```python
from build123d import *

# Parameters (mm, degrees)
BOSS_EXTRUDE1_DEPTH   = 8
CIRPATTERN1_COUNT     = 2
SKETCH3_R             = 12
CUT_EXTRUDE1_DEPTH    = 95.051900566
CUT_EXTRUDE2_START    = -2.6
CUT_EXTRUDE2_DEPTH    = 97.651900566
M3_CLEARANCE_HOLE1_D  = 3.4
CIRPATTERN2_COUNT     = 6
CIRPATTERN3_START     = 22
CIRPATTERN3_OUTLINE_R = 12
CIRPATTERN3_DEPTH     = 8
CUT_EXTRUDE3_DEPTH    = 3.6
M3_CLEARANCE_HOLE2_D  = 3.4
CIRPATTERN4_COUNT     = 6
SKETCH15_W            = 0.975112204
SKETCH15_H            = 3.233161508
CUT_EXTRUDE4_DEPTH    = 2.6
CIRPATTERN5_COUNT     = 3
CIRPATTERN5_ANGLE     = 120


# Read off the part's stored shape, not the designer's step: CSK for M3 Hex Socket Countersunk Cap Screw1, CirPattern3
with BuildPart() as part:
    # Sketch1 → Boss-Extrude1 (new body)
    with BuildSketch(Plane(origin=(0, 0, 0), x_dir=(1, 0, 0), z_dir=(0, 1, 0))):
        with BuildLine():
            Line((21.213203436, -21.213203436), (12.426406871, -30))
            Line((12.426406871, -30), (-54.826406871, -30))
            Line((-54.826406871, -30), (-54.826406871, -22))
            Line((-54.826406871, -22), (-23.763220436, 18.311454189))
            ThreePointArc((-23.763220436, 18.311454189), (19.803416038, 22.534966457), (21.213203436, -21.213203436))
        make_face()
    boss_extrude1 = extrude(amount=BOSS_EXTRUDE1_DEPTH)

    # CirPattern1: Boss-Extrude1 ×2 about axis
    cirpattern1_axis = Axis((-21.2, 15, 15), (0, 0.7071067811865476, -0.7071067811865476))
    for i in range(1, CIRPATTERN1_COUNT):
        add(boss_extrude1.rotate(cirpattern1_axis, i * 360 / CIRPATTERN1_COUNT))

    # Sketch3 → Cut-Extrude1 (cut, through all)
    with BuildSketch(Plane(origin=(0, 8, 0), x_dir=(1, 0, 0), z_dir=(0, 1, 0))):
        with Locations(Location((0, 0, 0), (0, 0, 270))):
            Circle(SKETCH3_R)
    extrude(amount=-CUT_EXTRUDE1_DEPTH, mode=Mode.SUBTRACT)

    # Sketch4 → Cut-Extrude2 (cut)
    with BuildSketch(Plane(origin=(0, 8, 0), x_dir=(1, 0, 0), z_dir=(0, 1, 0)).offset(CUT_EXTRUDE2_START)):
        Polygon((27, 3.233161507), (24.2, 1.616580754), (24.2, -1.616580754), (27, -3.233161507), (29.8, -1.616580754), (29.8, 1.616580754), align=None)
    cut_extrude2 = extrude(amount=CUT_EXTRUDE2_DEPTH, mode=Mode.SUBTRACT)

    # M3 Clearance Hole1 (through all)
    with Locations(Plane(origin=(0, 5.4, 0), x_dir=(1, 0, 0), z_dir=(0, 1, 0))):
        with Locations((27, 0)):
            m3_clearance_hole1 = Hole(M3_CLEARANCE_HOLE1_D / 2)

    # CirPattern2: Cut-Extrude2, M3 Clearance Hole1 ×6 about axis
    cirpattern2_axis = Axis((0, 0, 0), (0, 1, 0))
    add([cut_extrude2.rotate(cirpattern2_axis, i * 360 / CIRPATTERN2_COUNT) for i in range(1, CIRPATTERN2_COUNT)], mode=Mode.SUBTRACT)
    add([m3_clearance_hole1.rotate(cirpattern2_axis, i * 360 / CIRPATTERN2_COUNT) for i in range(1, CIRPATTERN2_COUNT)], mode=Mode.SUBTRACT)

    # CSK for M3 Hex Socket Countersunk Ca 2 → CSK for M3 Hex Socket Countersunk Cap Screw1 (revolve, cut)
    with BuildSketch(Plane(origin=(-15.5, 0, -15.5), x_dir=(1, 0, 0), z_dir=(0, 0, 1))):
        Polygon((1.8, 1.56), (1.8, 8), (0, 8), (0, 0), (3.36, 0), align=None)
    revolve(axis=Axis((-15.5, 0, -15.5), (0, 1, 0)), mode=Mode.SUBTRACT)

    # CSK for M3 Hex Socket Countersunk Ca 3 o → CSK for M3 Hex Socket Countersunk Ca 3 (revolve, cut)
    with BuildSketch(Plane(origin=(15.5, 0, 15.5), x_dir=(1, 0, 0), z_dir=(0, 0, 1))):
        Polygon((1.8, 1.56), (1.8, 8), (0, 8), (0, 0), (3.36, 0), align=None)
    revolve(axis=Axis((15.5, 0, 15.5), (0, 1, 0)), mode=Mode.SUBTRACT)

    # CSK for M3 Hex Socket Countersunk Ca 4 o → CSK for M3 Hex Socket Countersunk Ca 4 (revolve, cut)
    with BuildSketch(Plane(origin=(-15.5, 0, 15.5), x_dir=(1, 0, 0), z_dir=(0, 0, 1))):
        Polygon((1.8, 1.56), (1.8, 8), (0, 8), (0, 0), (3.36, 0), align=None)
    revolve(axis=Axis((-15.5, 0, 15.5), (0, 1, 0)), mode=Mode.SUBTRACT)

    # CSK for M3 Hex Socket Countersunk Ca 5 o → CSK for M3 Hex Socket Countersunk Ca 5 (revolve, cut)
    with BuildSketch(Plane(origin=(15.5, 0, -15.5), x_dir=(1, 0, 0), z_dir=(0, 0, 1))):
        Polygon((1.8, 1.56), (1.8, 8), (0, 8), (0, 0), (3.36, 0), align=None)
    revolve(axis=Axis((15.5, 0, -15.5), (0, 1, 0)), mode=Mode.SUBTRACT)

    # CirPattern3 outline → CirPattern3 (cut)
    with BuildSketch(Plane.XY.offset(CIRPATTERN3_START)):
        with Locations((-42.4, 30)):
            Circle(CIRPATTERN3_OUTLINE_R)
    extrude(amount=CIRPATTERN3_DEPTH, mode=Mode.SUBTRACT)

    # CirPattern3 2 outline → CirPattern3 2 (revolve, cut)
    with BuildSketch(Plane(origin=(-26.9, 45.5, 0), x_dir=(1, 0, 0), z_dir=(0, -1, 0))):
        Polygon((0, 22), (1.8, 22), (1.8, 28.44), (3.36, 30), (0, 30), align=None)
    revolve(axis=Axis((-26.9, 45.5, 0), (0, 0, 1)), mode=Mode.SUBTRACT)

    # CirPattern3 3 outline → CirPattern3 3 (revolve, cut)
    with BuildSketch(Plane(origin=(-57.9, 14.5, 0), x_dir=(1, 0, 0), z_dir=(0, -1, 0))):
        Polygon((0, 22), (1.8, 22), (1.8, 28.44), (3.36, 30), (0, 30), align=None)
    revolve(axis=Axis((-57.9, 14.5, 0), (0, 0, 1)), mode=Mode.SUBTRACT)

    # CirPattern3 4 outline → CirPattern3 4 (revolve, cut)
    with BuildSketch(Plane(origin=(-26.9, 14.5, 0), x_dir=(1, 0, 0), z_dir=(0, -1, 0))):
        Polygon((0, 22), (1.8, 22), (1.8, 28.44), (3.36, 30), (0, 30), align=None)
    revolve(axis=Axis((-26.9, 14.5, 0), (0, 0, 1)), mode=Mode.SUBTRACT)

    # CirPattern3 5 outline → CirPattern3 5 (revolve, cut)
    with BuildSketch(Plane(origin=(-57.9, 45.5, 0), x_dir=(1, 0, 0), z_dir=(0, -1, 0))):
        Polygon((0, 22), (1.8, 22), (1.8, 28.44), (3.36, 30), (0, 30), align=None)
    revolve(axis=Axis((-57.9, 45.5, 0), (0, 0, 1)), mode=Mode.SUBTRACT)

    # Sketch11 → Cut-Extrude3 (cut)
    with BuildSketch(Plane(origin=(0, 0, 22), x_dir=(-1, 0, 0), z_dir=(0, 0, -1))):
        Polygon((45.633161507, 46), (44.016580754, 48.8), (40.783419246, 48.8), (39.166838493, 46), (40.783419246, 43.2), (44.016580754, 43.2), align=None)
    cut_extrude3 = extrude(amount=-CUT_EXTRUDE3_DEPTH, mode=Mode.SUBTRACT)

    # M3 Clearance Hole2 (through all)
    with Locations(Plane(origin=(0, 0, 25.6), x_dir=(-1, 0, 0), z_dir=(0, 0, -1))):
        with Locations((42.4, 46)):
            m3_clearance_hole2 = Hole(M3_CLEARANCE_HOLE2_D / 2)

    # CirPattern4: Cut-Extrude3, M3 Clearance Hole2 ×6 about axis
    cirpattern4_axis = Axis((-42.4, 30, 0), (0, 0, 1))
    add([cut_extrude3.rotate(cirpattern4_axis, i * 360 / CIRPATTERN4_COUNT) for i in range(1, CIRPATTERN4_COUNT)], mode=Mode.SUBTRACT)
    add([m3_clearance_hole2.rotate(cirpattern4_axis, i * 360 / CIRPATTERN4_COUNT) for i in range(1, CIRPATTERN4_COUNT)], mode=Mode.SUBTRACT)

    # Sketch15 → Cut-Extrude4 (cut)
    with BuildSketch(Plane(origin=(0, 8, 0), x_dir=(1, 0, 0), z_dir=(0, 1, 0))):
        with Locations((30.287556102, 0)):
            Rectangle(SKETCH15_W, SKETCH15_H)
    cut_extrude4 = extrude(amount=-CUT_EXTRUDE4_DEPTH, mode=Mode.SUBTRACT)

    # CirPattern5: Cut-Extrude4 ×3 about axis
    cirpattern5_axis = Axis((0, 0, 0), (0, 1, 0))
    for i in range(1, CIRPATTERN5_COUNT):
        add(cut_extrude4.rotate(cirpattern5_axis, i * CIRPATTERN5_ANGLE / (CIRPATTERN5_COUNT - 1)), mode=Mode.SUBTRACT)


solid = part.part
```
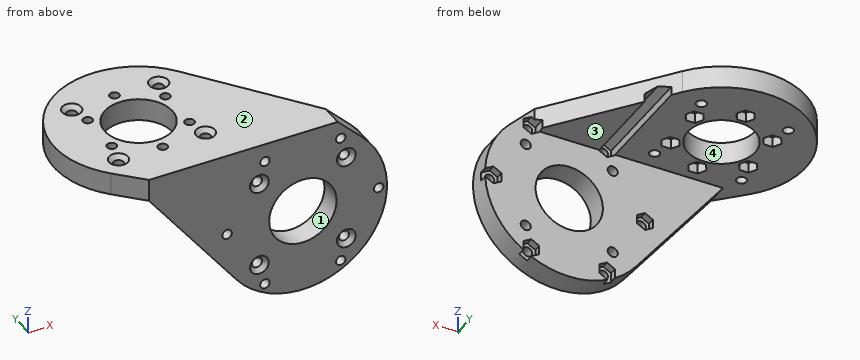
Geometry check sheet. Reference: the model listing, model coordinates, mm. Face numbers are marked on the shaded views. Give positions to 0.01 mm unless a question says otherwise; leave off trailing zeros. Write each loop counter-clockwise with the first axis right and the second up, starting at its lowest first coordinate (ties: lowest second). Pieces come first, ordered by that corner, then holes. Notation, with made-up numbers: (43.25, 29) -> (58.25, 29) arc R20 ccw to (58.25, 43) -> close; hole circle Ø10 at (-20, 20.25). An arc over 180 degrees is marked (long way). One line per question, with ' | ' between items.
Item 1: Draft check along Z on the marked faces 1, 2, 3 and 4. Enter one of: released by +Z, released by -Z, zero draft, split by the parting line, or undercut.
Determined:
face 1: undercut | face 2: released by +Z | face 3: released by -Z | face 4: zero draft
Item 2: Sectioned sample at B-B, the plane x = 5. Record the boundary of the cut face in (y, z), plus the area to 3 significant figures.
Determined:
outline: (0, -29.58) -> (8, -29.58) -> (8, -10.91) -> (0, -10.91) -> close; (0, 10.91) -> (8, 10.91) -> (8, 22) -> (17.64, 22) -> (17.64, 30) -> (0, 30) -> close | area: 379 mm^2
Item 3: Depth check by flat-ended pin: pin 1 (3 mm diameter, centred on y = 7, z = 0.5, fed in from -X); pin 2 (2.5 mm diameter, centred on x = -57, z = 23.5, fed in from -Y); pin 3 (4 mm diameter, centred on y = 9, z = -16, fed in from +X). Enter the tip coordinate at first touch or a pass-through.
Determined:
pin 1: x = -39.41 | pin 2: y = 0.92 | pin 3: x = 26.39
Item 4: Sectioned sample at C-C, the plane x = -42.4. Record the boundary of the cut face in (y, z).
Determined:
outline: (0, 5.87) -> (8, 5.87) -> (8, 22) -> (11.2, 22) -> (11.2, 25.6) -> (12.3, 25.6) -> (12.3, 30) -> (0, 30) -> close; (15.7, 25.6) -> (16.8, 25.6) -> (16.8, 22) -> (18, 22) -> (18, 30) -> (15.7, 30) -> close; (42, 22) -> (43.2, 22) -> (43.2, 25.6) -> (44.3, 25.6) -> (44.3, 30) -> (42, 30) -> close; (47.7, 25.6) -> (48.8, 25.6) -> (48.8, 22) -> (60, 22) -> (60, 30) -> (47.7, 30) -> close
Item 5: Scan lines: line 1 along Y through (x, z) = (-42.4, 28.9); line 2 along Z through (x, y) = (-15, 6); line 3 along Y through (x, z) = (-57.9, 25). Record each from-to range of solid material in increasing order.
Determined:
line 1: 0 to 12.3, 15.7 to 18, 42 to 44.3, 47.7 to 60 | line 2: -21.02 to -17.23, -13.77 to 13.77, 17.23 to 21.02, 25.75 to 30 | line 3: 3.07 to 12.7, 16.3 to 19.25, 24.75 to 35.25, 40.75 to 43.7, 47.3 to 55.69
Item 6: Sectioned sample at A-A, the plane z = 15.5. Record the boundary of the cut face in (x, y), plus the area to 3 significant figures.
Determined:
outline: (-49.82, 0) -> (-18.86, 0) -> (-17.3, 1.56) -> (-17.3, 8) -> (-49.82, 8) -> close; (-13.7, 1.56) -> (-12.14, 0) -> (12.14, 0) -> (13.7, 1.56) -> (13.7, 8) -> (-13.7, 8) -> close; (17.3, 1.56) -> (18.86, 0) -> (25.69, 0) -> (25.69, 8) -> (17.3, 8) -> close | area: 542 mm^2
